Can you work these out from the model? Positions are in its coordinate system, mm. Face numbers are marked on the shaded views. A direction names the side the tool comes from. Round coordinates to 2 decimals unless told otherwise and drop trailing zeros. Loops run counter-clockwise (first coordinate to the right, second up) from the corner with the lowest first, then second, coordinate; pieces in that order, holes last. Notation, with made-up numbers: M 52,-17 L 110,-17 A16 ccw 110,11 Z; hole C 15.5,88 d3. An arc over 180 degrees is marked long. Return JSON: item names as keys, results as strings.
```python
from build123d import *

# Parameters (mm, degrees)
SKETCH1_W               = 55
SKETCH1_H               = 55
BOSS_EXTRUDE1_DEPTH     = 10
SKETCH2_R               = 10
BOSS_EXTRUDE2_DEPTH     = 85
BOSS_EXTRUDE3_DEPTH     = 50
SKETCH4_R               = 7.5
CUT_EXTRUDE1_DEPTH      = 1
CUT_EXTRUDE1_DEPTH_BACK = 146
CUT_EXTRUDE2_REACH      = 49.5
SKETCH5_R               = 5
SKETCH5_R_2             = 3.5
SKETCH6_R               = 4.25
CUT_EXTRUDE3_DEPTH      = 50


with BuildPart() as part:
    # Sketch1 → Boss-Extrude1 (new body)
    with BuildSketch(Plane.XY):
        Rectangle(SKETCH1_W, SKETCH1_H)
    extrude(amount=BOSS_EXTRUDE1_DEPTH)

    # Sketch2 → Boss-Extrude2 (add)
    with BuildSketch(Plane.XY.offset(10)):
        Circle(SKETCH2_R)
    extrude(amount=BOSS_EXTRUDE2_DEPTH)

    # Sketch3 → Boss-Extrude3 (add)
    with BuildSketch(Plane.XY.offset(95)):
        with BuildLine():
            Line((-15, 0), (-15, 20))
            Line((-15, 20), (15, 20))
            Line((15, 20), (15, 0))
            ThreePointArc((15, 0), (0, -15), (-15, 0))
        make_face()
    extrude(amount=BOSS_EXTRUDE3_DEPTH)

    # Sketch4 → Cut-Extrude1 (cut, two sides)
    with BuildSketch(Plane(origin=(0, 0, 0), x_dir=(-1, 0, 0), z_dir=(0, 0, -1))) as cut_extrude1_sk:
        Circle(SKETCH4_R)
    extrude(amount=CUT_EXTRUDE1_DEPTH, mode=Mode.SUBTRACT)
    extrude(cut_extrude1_sk.sketch, amount=-CUT_EXTRUDE1_DEPTH_BACK, mode=Mode.SUBTRACT)

    # Sketch5 → Cut-Extrude2 (cut, up to next)
    with BuildSketch(Plane(origin=(0, 20, 0), x_dir=(1, 0, 0), z_dir=(0, 1, 0)), mode=Mode.PRIVATE) as cut_extrude2_sk1:
        with Locations((0, -135)):
            Circle(SKETCH5_R)
    cut_extrude2_tool1 = extrude(cut_extrude2_sk1.sketch, amount=-CUT_EXTRUDE2_REACH, mode=Mode.PRIVATE) & part.part
    add(cut_extrude2_tool1.solids().sort_by_distance((0, 20, 135))[0], mode=Mode.SUBTRACT)
    # Sketch5 → Cut-Extrude2 (cut, up to next)
    with BuildSketch(Plane(origin=(0, 20, 0), x_dir=(1, 0, 0), z_dir=(0, 1, 0)), mode=Mode.PRIVATE) as cut_extrude2_sk2:
        with Locations((0, -120)):
            Circle(SKETCH5_R_2)
    cut_extrude2_tool2 = extrude(cut_extrude2_sk2.sketch, amount=-CUT_EXTRUDE2_REACH, mode=Mode.PRIVATE) & part.part
    add(cut_extrude2_tool2.solids().sort_by_distance((0, 20, 120))[0], mode=Mode.SUBTRACT)
    # Sketch5 → Cut-Extrude2 (cut, up to next)
    with BuildSketch(Plane(origin=(0, 20, 0), x_dir=(1, 0, 0), z_dir=(0, 1, 0)), mode=Mode.PRIVATE) as cut_extrude2_sk3:
        with Locations((0, -105)):
            Circle(SKETCH5_R)
    cut_extrude2_tool3 = extrude(cut_extrude2_sk3.sketch, amount=-CUT_EXTRUDE2_REACH, mode=Mode.PRIVATE) & part.part
    add(cut_extrude2_tool3.solids().sort_by_distance((0, 20, 105))[0], mode=Mode.SUBTRACT)

    # Sketch6 → Cut-Extrude3 (cut)
    with BuildSketch(Plane.XY.offset(10)):
        with Locations((-19.5, 19.5)):
            Circle(SKETCH6_R)
        with Locations((19.5, 19.5)):
            Circle(SKETCH6_R)
        with Locations((19.5, -19.5)):
            Circle(SKETCH6_R)
        with Locations((-19.5, -19.5)):
            Circle(SKETCH6_R)
    extrude(amount=-CUT_EXTRUDE3_DEPTH, mode=Mode.SUBTRACT)


solid = part.part
```
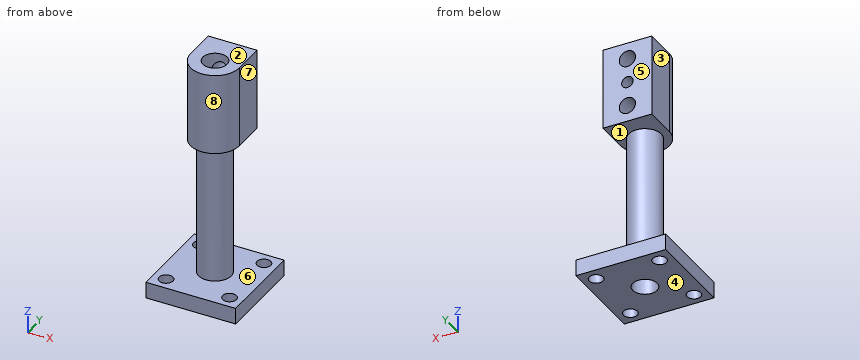
Q1. Suppose I cut it at A-A, the plane x = 19.5. Please give me the cut outline in (y, z).
Results:
{"outline": "M -27.5,0 L -23.75,0 L -23.75,10 L -27.5,10 Z; M -15.25,0 L 15.25,0 L 15.25,10 L -15.25,10 Z; M 23.75,0 L 27.5,0 L 27.5,10 L 23.75,10 Z"}
Q2. I'm going to push flat-ended pins straight in: pin 1 Ø4 at (x, z) = (4, 112) entering from -Y; pin 2 Ø6 at (y, z) = (11.5, 115) entering from +X; pin 3 Ø7 at (x, y) = (-19.5, -19.5) entering from -Z; pin 4 Ø1.5 at (y, z) = (-2, 125) entering from +X. Where does each tip first touch, or does it pass through?
Results:
{"pin 1": "stops at y = -14.87", "pin 2": "stops at x = 15", "pin 3": "passes through", "pin 4": "stops at x = 14.95"}
Q3. Thinking about a two-plate mould opening in Z: for the marked faces 1, 2 and 3, which applies, pulls with the +Z half, pulls with the -Z half, needs draft (parallel to the pull), parting line crosses it, or undercut?
Results:
{"face 1": "undercut", "face 2": "pulls with the +Z half", "face 3": "needs draft"}
Q4. On a 3-axis mill with a long thin cutter (end or side, diameter ignored), from which of +Z, -Z, +X, -X, +Y, -Y can I reach the whole of each face in a straight line? I mean the marked faces 4, 5, 6, 7 and 8. Say none if no direction works.
Results:
{"face 4": "-Z, +X, -X, +Y, -Y", "face 5": "+Z, +X, -X, +Y", "face 6": "none", "face 7": "+Z, +X, +Y, -Y", "face 8": "+Z, -Y"}
Q5. If I drill on line 1 along Y through (x, z) = (-19, 4); line 2 along Z through (x, y) = (0, 14); line 3 along Y through (x, z) = (0, 71), over which ranges is the centre line in solid material (lowest first)?
Results:
{"line 1": "y = -27.5 to -23.72, -15.28 to 15.28, 23.72 to 27.5", "line 2": "z = 0 to 10, 95 to 100, 110 to 116.5, 123.5 to 130, 140 to 145", "line 3": "y = -10 to -7.5, 7.5 to 10"}
Q6. Suppose I cut it at D-D, the plane y = -3. Please give me the cut outline in (x, z), plus the area to 3 significant figures.
Results:
{"outline": "M -27.5,0 L -6.87,0 L -6.87,145 L -14.7,145 L -14.7,95 L -9.54,95 L -9.54,10 L -27.5,10 Z; M 6.87,0 L 27.5,0 L 27.5,10 L 9.54,10 L 9.54,95 L 14.7,95 L 14.7,145 L 6.87,145 Z", "area": "1,650 mm2"}
Q7. Suppose I cut it at C-C, the plane z = 120. Please give me the cut outline in (x, y), plus the area to 3 significant figures.
Results:
{"outline": "M -15,0 A15 ccw 15,0 L 15,20 L 3.5,20 L 3.5,6.63 A7.5 cw long -3.5,6.63 L -3.5,20 L -15,20 Z", "area": "687 mm2"}
